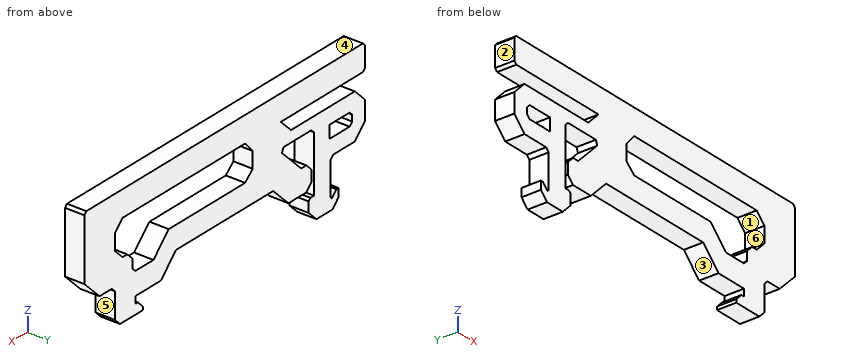
Autodesk Inventor part; units mm, degrees
ref_plane "YZ Plane" through (0, 0, 0) normal (1, 0, 0) x (0, 1, 0)
ref_plane "XZ Plane" through (0, 0, 0) normal (0, 1, 0) x (-1, 0, 0)
ref_plane "XY Plane" through (0, 0, 0) normal (0, 0, 1) x (1, 0, 0)
sketch "Sketch1" plane through (0, 0, 0) normal (0, 1, 0) x (-1, 0, 0)
  line L0 (-17.6312, -19.1085) -> (1.2602, -19.1085)
  line L1 (-32.5455, -19.1086) -> (-30.1592, -19.1086)
  line L2 (-33.9375, -17.7166) -> (-32.5455, -19.1086)
  line L3 (-35.5284, -16.1257) -> (-33.9375, -17.7166)
  line L4 (2.9824, -14.5915) -> (3.2737, -13.8887)
  line L5 (-2.717, -14.3021) -> (-4.2084, -15.6146)
  line L6 (-2.717, -11.8304) -> (-4.2084, -10.16)
  line L7 (18.7576, -6.1828) -> (-35.133, -6.1828)
  line L8 (18.7597, -10.1584) -> (2.7517, -10.1584)
  line L9 (-29.5627, -14.1232) -> (-28.0713, -15.6146)
  line L10 (18.7576, -6.1828) -> (19.157, -6.5801)
  line L11 (19.157, -6.5801) -> (19.157, -9.7618)
  line L12 (19.157, -9.7618) -> (18.7597, -10.1584)
  line L13 (2.7517, -10.1584) -> (4.7402, -12.147)
  line L14 (4.7402, -12.147) -> (17.1688, -12.147)
  line L15 (17.1688, -12.147) -> (19.1574, -14.1355)
  line L16 (19.1574, -14.1355) -> (19.1574, -17.1184)
  line L17 (19.1574, -17.1184) -> (17.1688, -19.107)
  line L18 (17.1688, -19.107) -> (12.9431, -19.107)
  line L19 (12.9431, -19.107) -> (12.4459, -19.6041)
  line L20 (12.4459, -19.6041) -> (12.4459, -24.8441)
  line L21 (12.4459, -24.8441) -> (12.6845, -25.0822)
  line L22 (12.6845, -25.0822) -> (13.5894, -24.1758)
  line L23 (13.5894, -24.1758) -> (13.9871, -24.1758)
  line L24 (13.9871, -24.1758) -> (13.9871, -25.4685)
  line L25 (13.9871, -25.4685) -> (12.7939, -26.6636)
  line L26 (12.7939, -26.6636) -> (9.7117, -26.6636)
  line L27 (9.7117, -26.6636) -> (8.1705, -25.1225)
  line L28 (8.1705, -23.5316) -> (8.1705, -25.1225)
  line L29 (8.5185, -23.1836) -> (9.2145, -23.1836)
  line L30 (2.9824, -14.5915) -> (6.7288, -18.3379)
  line L31 (6.7288, -18.3379) -> (7.7231, -18.3379)
  line L32 (7.7231, -18.3379) -> (8.7174, -19.3322)
  line L33 (8.7174, -19.3322) -> (8.7174, -21.097)
  line L34 (8.7174, -21.097) -> (7.7231, -22.0913)
  line L35 (7.7231, -22.0913) -> (4.2431, -22.0913)
  line L36 (4.2431, -22.0913) -> (1.2602, -19.1085)
  line L37 (-17.6312, -19.1085) -> (-20.6141, -22.0913)
  line L38 (-20.6141, -22.0913) -> (-25.5855, -22.0913)
  line L39 (-25.5855, -22.0913) -> (-25.5855, -23.1851)
  line L40 (-25.5855, -23.1851) -> (-25.0884, -23.1851)
  line L41 (-25.0884, -23.1851) -> (-24.0941, -24.1794)
  line L42 (-24.0941, -24.1794) -> (-24.0941, -24.6766)
  line L43 (-24.0941, -24.6766) -> (-28.5683, -24.6766)
  line L44 (-28.5683, -24.6766) -> (-29.5626, -23.6823)
  line L45 (-29.5626, -23.6823) -> (-29.5626, -19.7051)
  line L46 (-29.5626, -19.7051) -> (-30.1592, -19.1086)
  line L47 (-35.5284, -16.1257) -> (-35.5284, -6.5807)
  line L48 (-35.5284, -6.5807) -> (-35.133, -6.1828)
  line L49 (-29.5627, -14.1232) -> (-29.5627, -11.6514)
  line L50 (-29.5627, -11.6514) -> (-28.0713, -10.16)
  line L51 (-28.0713, -10.16) -> (-4.2084, -10.16)
  line L52 (-2.717, -11.8304) -> (-2.717, -14.3021)
  line L53 (-4.2084, -15.6146) -> (-19.0784, -15.6146)
  line L54 (-22.0613, -18.5974) -> (-25.5855, -18.5974)
  line L55 (-26.1821, -16.6089) -> (-27.1764, -15.6146)
  line L56 (-26.1821, -18.0009) -> (-26.1821, -16.6089)
  line L57 (-27.1764, -15.6146) -> (-28.0713, -15.6146)
  line L58 (-25.5855, -18.5974) -> (-26.1821, -18.0009)
  line L59 (-19.0784, -15.6146) -> (-22.0613, -18.5974)
  line L60 (12.211, -16.6077) -> (12.211, -14.6465)
  line L61 (12.211, -14.6465) -> (16.1607, -14.6465)
  line L62 (16.1607, -14.6465) -> (16.6579, -15.1437)
  line L63 (16.6579, -15.1437) -> (16.6579, -16.1106)
  line L64 (16.6579, -16.1106) -> (16.1607, -16.6077)
  line L65 (16.1607, -16.6077) -> (12.211, -16.6077)
  line L66 (8.5185, -23.1836) -> (8.1705, -23.5316)
  line L67 (9.2145, -14.3859) -> (9.2145, -23.1836)
  line L68 (8.7174, -13.8887) -> (9.2145, -14.3859)
  line L69 (8.7174, -13.8887) -> (3.2737, -13.8887)
  point P0 (0, 0)
  point P1 (-29.5627, -12.8873)
  dimension "d2" = 9.545
  dimension "d3" = 3.9771
  dimension "d4" = 4.4743
  dimension "d6" = 4.9714
  dimension "d7" = 3.5242
  dimension "d9" = 2.9829
  dimension "d11" = 0.9943
  dimension "d12" = 0.398
  dimension "d13" = 53.8907
  dimension "d14" = 2.4718
  dimension "d15" = 1.4914
  dimension "d16" = 1.4914
  dimension "d18" = 1.392
  dimension "d19" = 0.5966
  dimension "d20" = 23.8629
  dimension "d21" = 1.4914
  dimension "d22" = 2.4718
  dimension "d23" = 14.8701
  dimension "d24" = 2.9829
  dimension "d25" = 18.8914
  dimension "d27" = 2.9829
  dimension "d28" = 2.9829
  dimension "d29" = 3.48
  dimension "d30" = 3.7464
  dimension "d31" = 0.7028
  dimension "d32" = 5.4437
  dimension "d33" = 8.7978
  dimension "d34" = 0.4971
  dimension "d35" = 1.5909
  dimension "d36" = 0.348
  dimension "d37" = 0.696
  dimension "d38" = 1.5411
  dimension "d39" = 3.0823
  dimension "d40" = 1.1931
  dimension "d41" = 1.2927
  dimension "d42" = 0.3977
  dimension "d43" = 0.9048
  dimension "d44" = 0.2386
  dimension "d45" = 5.24
  dimension "d46" = 0.4971
  dimension "d47" = 4.2257
  dimension "d48" = 1.9886
  dimension "d49" = 2.9829
  dimension "d50" = 1.9886
  dimension "d51" = 12.4286
  dimension "d52" = 1.9886
  dimension "d54" = 16.008
  dimension "d55" = 0.3973
  dimension "d56" = 3.1817
  dimension "d58" = 2.9829
  dimension "d59" = 2.9829
  dimension "d60" = 2.9829
  dimension "d61" = 0.9943
  dimension "d62" = 0.9943
  dimension "d63" = 0.9943
  dimension "d64" = 3.7463
  dimension "d66" = 1.7649
  dimension "d67" = 0.9943
  dimension "d68" = 0.9943
  dimension "d69" = 0.4971
  dimension "d75" = 0.4971
  dimension "d76" = 0.4971
  dimension "d77" = 0.4971
  dimension "d78" = 0.4971
extrude "Extrusion1" add sketch "Sketch1" along normal blind 3
properties part number "CO_1_01_dinRail"
CAD build for the part. Positions are in the model's coordinates, mm. Face numbers are marked on the shaded views. A direction names the side the tool comes from. Round coordinates to 2 decimals unless told otherwise and drop trailing zeros. Write each loop counter-clockwise with the first axis right and the second up, starting at its lowest first coordinate (ties: lowest second). Pieces come first, ordered by that corner, then holes. Notation, with made-up numbers: (13, 72.25) - (49, 72.25) arc R16 cw to (49, 100.25) - close; hole circle Ø9 at (85.25, 77). An arc over 180 degrees is marked (long way). Return JSON: item names as keys, results as strings. Group by question number.
Item 1: 3-axis set-ups, long thin cutter, end or side, ignore diameter. For the marked faces 1, 2 and 3: which of +Z, -Z, +X, -X, +Y, -Y reach the whole face in a straight line?
Item 2: Band-saw the part on A-A on x = 16. List the corners of the cut face in (y, z).
Item 3: Band-saw the part on C-C on x = 31. List the corners of the cut face in (y, z), plus the area to 3 significant figures.
Item 4: Band-saw the part on D-D on x = -2. List the corners of the cut face in (y, z).
Item 5: Flat gauge pins, fed straight in: pin 1 Ø1.5 at (x, y) = (-15.5, 1) entering from -Z; pin 2 Ø1.5 at (y, z) = (2, -20.5) entering from +X; pin 3 Ø1.5 at (y, z) = (1, -22.5) entering from -X. Where does each tip first touch, or does it go through?
Item 6: Probe probe 1 along Z at (x, y) = (-15.5, 0.15); probe 2 along Z at (x, y) = (7.5, 0.2); probe 3 along Z at (x, y) = (-13.5, 0.75). List the from-to ranges inside material, lowest first.
Item 7: Band-saw the part on B-B on y = 1.45. State how many separate pieces and enclosed holes the cut face has, plus the area to 3 significant figures.
Item 8: Mould opens along Z. For the marked faces 4, 5 and 6 say: +Z half, -Z half, draft (parallel to the pull), parting line (faces both ways), or undercut.
Resolved:
{
 "1": {"face 1": "+Y, -Y", "face 2": "+Z, -Z, -X, +Y, -Y", "face 3": "-Z, +Y, -Y"},
 "2": {"outline": "(0, -19.11) - (3, -19.11) - (3, -15.61) - (0, -15.61) - close; (0, -10.16) - (3, -10.16) - (3, -6.18) - (0, -6.18) - close"},
 "3": {"outline": "(0, -19.11) - (3, -19.11) - (3, -6.18) - (0, -6.18) - close", "area": "38.8 mm²"},
 "4": {"outline": "(0, -19.85) - (3, -19.85) - (3, -6.18) - (0, -6.18) - close"},
 "5": {"pin 1": "stops at z = -19.11", "pin 2": "stops at x = 29.56", "pin 3": "stops at x = -12.45"},
 "6": {"probe 1": "z = -19.11 to -16.61, -14.65 to -12.15, -10.16 to -6.18", "probe 2": "z = -19.11 to -15.61, -10.16 to -6.18", "probe 3": "z = -25.96 to -24.27, -19.11 to -16.61, -14.65 to -12.15, -10.16 to -6.18"},
 "7": {"separate pieces": "1", "enclosed holes": "2", "area": "568 mm²"},
 "8": {"face 4": "+Z half", "face 5": "draft", "face 6": "undercut"}
}
